Can you work these out from the model? Positions are in its coordinate system, mm. A direction names the side the tool comes from. Round coordinates to 2 decimals unless told otherwise and drop trailing zeros. Order: outer loops, then holes, each group sorted by start corner. A loop starts at its lowest first (then second) coordinate and runs counter-clockwise, first axis right, second up.
from build123d import *

# Parameters (mm, degrees)
CIRPATTERN1_COUNT = 16


with BuildPart() as part:
    # Sketch1 → Revolve1 (revolve)
    with BuildSketch(Plane.XY):
        Polygon((-76.2, -12.7), (-76.2, -31.75), (-42.8625, -31.75), (-15.875, -19.05), (0, -19.05), (0, 0), (-25.4, 0), (-50.8, -12.7), align=None)
    revolve(axis=Axis((0, -19.05, 0), (0, 1, 0)))

    # Sketch5 → 5/16 (0.3125) Diameter Hole1 (revolve, cut)
    with BuildSketch(Plane(origin=(-69.85, -12.7, 0), x_dir=(0, 0, 1), z_dir=(1, 0, 0))):
        Polygon((0, 0), (0, 40.484665582), (3.96875, 38.1), (3.96875, 0), align=None)
    f_5_16_0_3125_diameter_hole1 = revolve(axis=Axis((-69.85, -6.35, 0), (0, -1, 0)), mode=Mode.SUBTRACT)

    # CirPattern1: 5/16 (0.3125) Diameter Hole1 ×16 about axis
    cirpattern1_axis = Axis((0, 0, 0), (0, 1, 0))
    for i in range(1, CIRPATTERN1_COUNT):
        add(f_5_16_0_3125_diameter_hole1.rotate(cirpattern1_axis, i * 360 / CIRPATTERN1_COUNT), mode=Mode.SUBTRACT)

    # Sketch8 → 1/2 NPT Tapped Hole1 (revolve, cut)
    with BuildSketch(Plane(origin=(0, 0, 0), x_dir=(0, 0, 1), z_dir=(1, 0, 0))):
        Polygon((0, 0), (0, 19.05), (8.9281, 19.05), (8.9281, 13.462), (9.479726792, 13.462), (9.8827971, 0), align=None)
    revolve(axis=Axis((0, 6.35, 0), (0, -1, 0)), mode=Mode.SUBTRACT)


solid = part.part
(1) If we mould it in two halves opening along Z, with no side actions, what happens to faces 1 (the face through (-60.58, -22.09, 27.07)), 2 (the face through (-33, -31.75, -33)), 3 (the face through (60.47, -22.358, -46.367))? For each: pulls with the +Z half, pulls with the -Z half, needs draft (parallel to the pull), parting line crosses it, or undercut.
(2) I'm going to push flat-ended pins straight in: pin 1 Ø5 at (x, y) = (52.5, -25) entering from -Z; pin 2 Ø8 at (y, z) = (-11, -38) entering from -X; pin 3 Ø9.5 at (x, z) = (-5.5, -3.5) entering from -Y. Where does each tip first touch, or does it pass through?
(3) On a 3-axis mill with a long thin cutter (end or side, diameter ignored), from which of +Z, -Z, +X, -X, +Y, -Y can I reach the whole of each face in a straight line? I mean faces 4 (the face through (65.976, -22.092, 0.86)), 5 (the face through (6, -13.462, -7)), 6 (the face through (-7, -19.05, -7)). Say none if no direction works.
(4) I want a section at D-D, the plane x = 56.5. List the corners of the cut face in (y, z) for me.
(5) I want a section at A-A, the plane y = -30. Give the number of separate pieces and of enclosed holes in the cut face, plus the area to 3 significant figures.
(6) Please list where these lines run through material, in increasing order: probe 1 along Z at (x, y) = (0, -16.4); probe 2 along Z at (x, y) = (0, -23); probe 3 along X at (y, z) = (-22.5, 49).
(7) I want a section at B-B, the plane y = -3. List the corners of the cut face in (x, z) for me.
Ans:
1. face 1: undercut
1. face 2: needs draft
1. face 3: parting line crosses it
2. pin 1: stops at z = -57.5
2. pin 2: stops at x = -68
2. pin 3: stops at y = -19.05
3. face 4: +Y, -Y
3. face 5: +Y
3. face 6: -Y
4. outline: (-31.75, -51.13) - (-12.7, -51.13) - (-12.7, 51.13) - (-31.75, 51.13) - close
5. separate pieces: 1
5. enclosed holes: 17
5. area: 12,600 mm2
6. probe 1: z = -76.2 to -73.82, -65.88 to -8.93, 8.93 to 65.88, 73.82 to 76.2
6. probe 2: z = -76.2 to -73.82, -65.88 to -24.27, 24.27 to 65.88, 73.82 to 76.2
6. probe 3: x = -58.36 to -53.34, -45.44 to 45.44, 53.34 to 58.36
7. outline: circle Ø62.8 at (0, 0); hole circle Ø19.59 at (0, 0)
